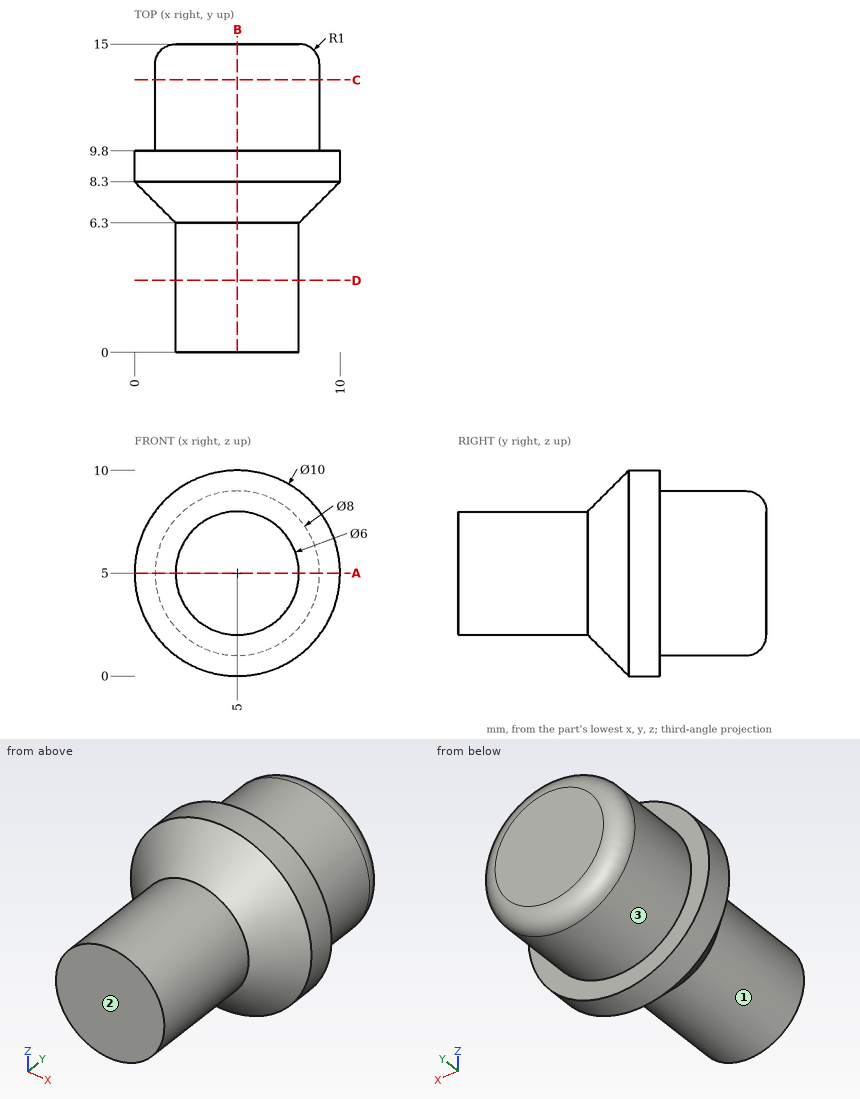
Print and shaded views of the part. All mm, measured from the part's lowest x, y and z. A direction names the side the tool comes from. Give positions to 0.01 mm unless a question says otherwise; leave off trailing zeros. Loops run counter-clockwise (first coordinate to the right, second up) from the corner with the lowest first, then second, coordinate; pieces in that order, holes last.
1) Saw through at B-B (x = 5). Write the cut outline in (y, z).
2) Wall check: line 1 (Z direction, x = 1, y = 9.75); line 2 (X direction, y = 11.25, z = 8); line 3 (Z direction, x = 2.25, y = 14.25). Give the ranges that are in metal, low to high.
3) Saw through at C-C (y = 13.25). Write the cut outline in (x, z).
4) Flat gauge pins, fed straight in: pin 1 Ø4 at (x, y) = (5.5, 10.5) entering from -Z; pin 2 Ø1.5 at (y, z) = (4, 3.5) entering from -X; pin 3 Ø1 at (y, z) = (13, 3) entering from -X. Where does each tip first touch, or does it go through?
5) Tool access for the marked faces 1, 2 and 3: list every direction of +Z, -Z, +X, -X, +Y, -Y with a clear straight run to the whole face (end or side of a thin tool).
6) Saw through at A-A (z = 5). Write the cut outline in (x, y).
7) Saw through at D-D (y = 3.5). Write the cut outline in (x, z).
Answer block:
1. outline: (0, 2) - (6.3, 2) - (8.3, 0) - (9.8, 0) - (9.8, 1) - (14, 1) arc R1 ccw to (15, 2) - (15, 8) arc R1 ccw to (14, 9) - (9.8, 9) - (9.8, 10) - (8.3, 10) - (6.3, 8) - (0, 8) - close
2. line 1: z = 2 to 8
2. line 2: x = 2.35 to 7.65
2. line 3: z = 2.14 to 7.86
3. outline: circle Ø8 at (5, 5)
4. pin 1: stops at z = 0
4. pin 2: stops at x = 2.1
4. pin 3: stops at x = 1.29
5. face 1: -Y
5. face 2: +Z, -Z, +X, -X, -Y
5. face 3: +Y
6. outline: (0, 8.3) - (2, 6.3) - (2, 0) - (8, 0) - (8, 6.3) - (10, 8.3) - (10, 9.8) - (9, 9.8) - (9, 14) arc R1 ccw to (8, 15) - (2, 15) arc R1 ccw to (1, 14) - (1, 9.8) - (0, 9.8) - close
7. outline: circle Ø6 at (5, 5)
